Verification items for this drawing (mm, ordinates from the low corner). Give positions to 0.01 mm unless a question says otherwise; leave off trailing zeros. Write each loop counter-clockwise with the first axis right and the second up, starting at its lowest first coordinate (ties: lowest second). Pieces come first, ordered by that corner, then holes. Notation, with made-up numbers: (78, -23) -> (119, -23) arc R20 ccw to (119, -11) -> close; hole circle Ø11 at (-38, 6). An arc over 180 degrees is marked (long way). One line per item, written item: value.
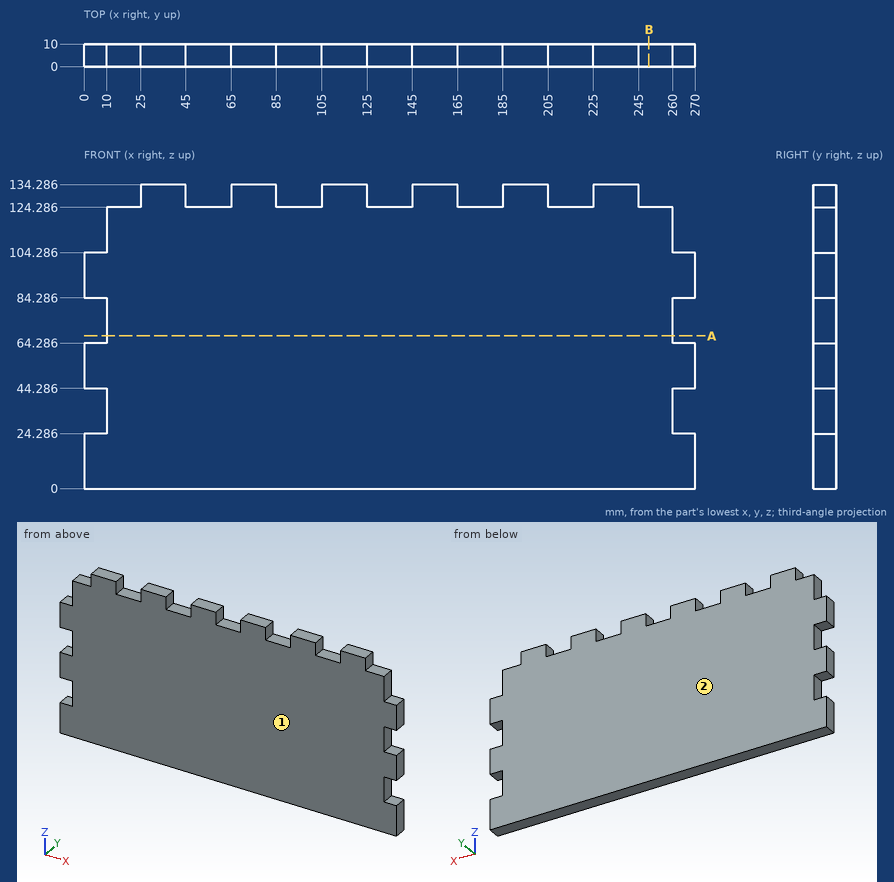
1) Mould release check, pull along Y, two halves, no side actions. Record for the marked faces 1 and 2: released by +Y, released by -Y, zero draft, split by the parting line, or undercut.
Verdict:
face 1: released by -Y
face 2: released by +Y
2) Depth check by flat-ended pin: pin 1 Ø3 at (y, z) = (5, 118) entering from +X; pin 2 Ø5 at (x, y) = (6, 4) entering from +Z; pin 3 Ø3 at (y, z) = (4.5, 76.5) entering from -X. Enter the tip coordinate at first touch or a pass-through.
Verdict:
pin 1: x = 260
pin 2: z = 104.29
pin 3: x = 10
3) Sectioned sample at B-B on x = 249.5. Record the cut outline in (y, z).
Verdict:
outline: (0, 0) -> (10, 0) -> (10, 124.29) -> (0, 124.29) -> close
4) Sectioned sample at A-A on z = 67.5. Record the cut outline in (x, y).
Verdict:
outline: (10, 0) -> (260, 0) -> (260, 10) -> (10, 10) -> close
5) Scan lines: probe 1 along Z at (x, y) = (17, 8.75); probe 2 along X at (y, z) = (8.25, 32.5). Record each from-to range of solid material in increasing order.
Verdict:
probe 1: 0 to 124.29
probe 2: 10 to 260
